Geometry: final body of the model. Coordinates: model frame, mm. A direction names the side the tool comes from. Give positions to 0.01 mm unless a question says otherwise; leave off trailing zeros. Write each loop counter-clockwise with the first axis right and the second up, starting at its lowest first coordinate (ties: lowest second). Pieces come first, ordered by that corner, then holes.
Autodesk Inventor part; units mm, degrees
ref_plane "YZ Plane" through (0, 0, 0) normal (1, 0, 0) x (0, 1, 0)
ref_plane "XZ Plane" through (0, 0, 0) normal (0, 1, 0) x (-1, 0, 0)
ref_plane "XY Plane" through (0, 0, 0) normal (0, 0, 1) x (1, 0, 0)
sketch "Skizze1" plane through (0, 0, 0) normal (0, 0, 1) x (1, 0, 0)
  line L0 (-60, 0) -> (60, 0)
  line L1 (60, 0) -> (60, 20)
  line L2 (60, 20) -> (45, 20)
  line L3 (45, 20) -> (45, 54)
  line L4 (38.5, 70) -> (-50.5, 70)
  line L5 (-60, 41) -> (-60, 0)
  line L6 (-60, 57) -> (-60, 44)
  line L7 (-60, 44) -> (-63, 44)
  line L8 (-63, 44) -> (-63, -3)
  line L9 (-63, -3) -> (63, -3)
  line L10 (63, -3) -> (63, 23)
  line L11 (63, 23) -> (48, 23)
  line L12 (48, 23) -> (48, 57)
  line L13 (41.5, 73) -> (-53.5, 73)
  line L14 (-60, 41) -> (-57, 41)
  line L15 (-57, 54) -> (-50.5, 54)
  line L16 (-50.5, 54) -> (-50.5, 70)
  line L17 (-60, 57) -> (-53.5, 57)
  line L18 (-53.5, 73) -> (-53.5, 57)
  line L19 (-57, 54) -> (-57, 41)
  line L20 (-50.5, 70) -> (-40.5, 70)
  line L21 (-40.5, 70) -> (-40.5, 65)
  line L22 (-40.5, 65) -> (-50.5, 65)
  line L23 (-50.5, 65) -> (-50.5, 70)
  line L24 (10.5, 70) -> (15.5, 70)
  line L25 (15.5, 70) -> (15.5, 65)
  line L26 (15.5, 65) -> (10.5, 65)
  line L27 (10.5, 65) -> (10.5, 70)
  line L28 (41.5, 73) -> (41.5, 57)
  line L29 (41.5, 57) -> (48, 57)
  line L30 (38.5, 70) -> (38.5, 54)
  line L31 (38.5, 54) -> (45, 54)
  line L32 (-60, 0) -> (-52, 0)
  line L33 (-52, 0) -> (-52, 6)
  line L34 (-52, 6) -> (-60, 6)
  line L35 (-60, 6) -> (-60, 0)
  line L36 (24.5, 6) -> (31.5, 6)
  line L37 (31.5, 6) -> (31.5, 0)
  line L38 (31.5, 0) -> (24.5, 0)
  line L39 (24.5, 0) -> (24.5, 6)
  line L40 (-57, 41) -> (-60, 41)
  line L41 (-60, 41) -> (-60, 6)
  line L42 (-60, 6) -> (-57, 6)
  line L43 (-57, 6) -> (-57, 41)
  line L44 (-50.5, 59.5) -> (38.5, 59.5)
  line L45 (-50.5, 59.5) -> (-50.5, 65)
  line L46 (-50.5, 65) -> (-40.5, 65)
  line L47 (-40.5, 65) -> (-40.5, 70)
  line L48 (-40.5, 70) -> (10.5, 70)
  line L49 (10.5, 70) -> (10.5, 65)
  line L50 (10.5, 65) -> (15.5, 65)
  line L51 (15.5, 65) -> (15.5, 70)
  line L52 (15.5, 70) -> (38.5, 70)
  line L53 (38.5, 70) -> (38.5, 59.5)
  point P0 (0, 0)
  point P1 (41.5, 70)
  point P2 (0, 0)
  dimension "d0" = 120
  dimension "d9" = 15
  dimension "d13" = 70
  dimension "d17" = 3
  dimension "d18" = 3
  dimension "d19" = 3
  dimension "d20" = 3
  dimension "d30" = 3
  dimension "d31" = 20
  dimension "d32" = 41
  dimension "d37" = 3
  dimension "d38" = 54
  dimension "d39" = 3
  dimension "d41" = 3
  dimension "d43" = 3
  dimension "d47" = 10
  dimension "d48" = 5
  dimension "d49" = 51
  dimension "d50" = 3
  dimension "d51" = 3
  dimension "d52" = 89
  dimension "d53" = 8
  dimension "d54" = 6
  dimension "d55" = 8
  dimension "d58" = 3
  dimension "d59" = 3
  dimension "d60" = 7
  dimension "d61" = 76.5
  dimension "d68" = 5.5
extrude "Extrusion1" add sketch "Skizze1" along normal blind 150 contours L16 L4 L21 L22 | L25 L26 L27 L4 | L17 L18 L13 L28 L29 L12 L11 L10 L9 L8 L7 L6
extrude "Extrusion3" add sketch "Skizze1" along normal blind 133 contours L5 L34 L33 L0 | L5 L14 L43 L34
sketch "Skizze3" plane through (-53.5, 73, 0) normal (0, 1, 0) x (1, 0, 0)
  line L0 (13, -62) -> (64, -62)
  line L1 (64, -62) -> (64, -150)
  line L2 (64, -150) -> (13, -150)
  line L3 (13, -150) -> (13, -62)
  line L4 (0, 0) -> (0, -150)
  line L5 (95, -150) -> (0, -150)
  point P0 (60, 0)
  dimension "d25" = 51
  dimension "d26" = 88
  dimension "d45" = 13
extrude "Extrusion2" cut sketch "Skizze3" against normal up to surface (3 mm away)
extrude "Extrusion5" add sketch "Skizze1" along normal blind 55 contours L16 L22 L21 L4 L27 L26 L25 L30 L44
equation "\"d18\" = d20"
equation "\"d19\" = d20"
equation "\"d30\" = d20"
equation "\"d37\" = d20"
equation "\"d39\" = d20"
equation "\"d41\" = d20"
equation "\"d43\" = d20"
equation "\"d50\" = d20"
equation "\"d51\" = d20"
equation "\"d58\" = d20"
properties part number "Gehäuse"
Q1. Pull-direction query (X, two-part tool) for faces 4 (the flat face through (-50.5, 59, 91)), 5 (the flat face through (41.5, 65, 74)), 6 (the flat face through (-5, 73, 57)), 7 (the flat face through (-45, 65, 102)); classes: released by +X, released by -X, zero draft, split by the parting line, or undercut.
Filled sheet:
face 4: undercut
face 5: released by +X
face 6: zero draft
face 7: undercut
Q2. Ray query, line 1 along X through (y, z) = (68.5, 131); line 2 along X through (y, z) = (12, 97.5); line 3 along X through (y, z) = (49, 47). Return the intervals inside material, ascending.
Filled sheet:
line 1: x = -53.5 to -40.5, 10.5 to 15.5, 38.5 to 41.5
line 2: x = -63 to -57, 60 to 63
line 3: x = -60 to -57, 45 to 48
Q3. Access query for faces 1 (the flat face through (-15, 70, 58)), 2 (the flat face through (-52, 3, 66)), 3 (the flat face through (-60, 51, 74)). Directions: +Z, -Z, +X, -X, +Y, -Y. A direction counts if a zero-diameter tool reaches every point of the face in a straight line with its end or side. Return the directions, or none.
Filled sheet:
face 1: +Z
face 2: +Z, -Z
face 3: +Z, -Z, -X, +Y
Q4. Pin query (flat end, axial travel): P1, Ø1.5, axis at y = 67.5, z = 90, coming from the +X side; P2, Ø1.5, axis at x = -21.5, y = 71.5, coming from the +Z side; P3, Ø10, axis at x = -38, y = 58.5, coming from the +Z side. Return the tip coordinate at first contact, or that it passes through.
Filled sheet:
P1: stops at x = 41.5
P2: stops at z = 62
P3: stops at z = 55
Q5. Section B-B on x = 3. Output: boundary loops of the cut face in (y, z), plus the area to 3 significant figures.
Filled sheet:
outline: (-3, 0) - (0, 0) - (0, 150) - (-3, 150) - close; (59.5, 0) - (73, 0) - (73, 62) - (70, 62) - (70, 55) - (59.5, 55) - close
area: 1,210 mm2
Q6. Section A-A on y = 49.5. Output: boundary loops of the cut face in (x, z).
Filled sheet:
outline: (-60, 0) - (-57, 0) - (-57, 150) - (-60, 150) - close; (45, 0) - (48, 0) - (48, 150) - (45, 150) - close
Q7. Section D-D on y = 11. Output: boundary loops of the cut face in (x, z).
Filled sheet:
outline: (-63, 0) - (-57, 0) - (-57, 133) - (-60, 133) - (-60, 150) - (-63, 150) - close; (60, 0) - (63, 0) - (63, 150) - (60, 150) - close
